from build123d import *

# Parameters (mm, degrees)
FILLET2_R               = 8
FILLET3_R               = 6
FILLET4_R               = 6
SKETCH3_R               = 10
CUT_EXTRUDE2_DEPTH      = 10
CUT_EXTRUDE2_DEPTH_BACK = 121
CHAMFER2_SIZE           = 6


with BuildPart() as part:
    # Sketch2 → Revolve1 (revolve)
    with BuildSketch(Plane.XY):
        Polygon((10, 120), (10, 0), (100, 0), (100, 20), (60, 20), (60, 60), (40, 60), (40, 120), align=None)
    revolve(axis=Axis((10, 120, 0), (0, -1, 0)))

    # Fillet2
    fillet2_edges = [part.edges().sort_by_distance(p)[0] for p in [
        (-80, 20, 0),
    ]]
    fillet(fillet2_edges, radius=FILLET2_R)

    # Fillet3
    fillet3_edges = [part.edges().sort_by_distance(p)[0] for p in [
        (-40, 20, 0),
    ]]
    fillet(fillet3_edges, radius=FILLET3_R)

    # Fillet4
    fillet4_edges = [part.edges().sort_by_distance(p)[0] for p in [
        (-20, 60, 0),
    ]]
    fillet(fillet4_edges, radius=FILLET4_R)

    # Sketch3 → Cut-Extrude2 (cut, two sides)
    with BuildSketch(Plane(origin=(0, 120, 0), x_dir=(1, 0, 0), z_dir=(0, 1, 0))) as cut_extrude2_sk:
        with Locations((10, 0)):
            Circle(SKETCH3_R)
    extrude(amount=CUT_EXTRUDE2_DEPTH, mode=Mode.SUBTRACT)
    extrude(cut_extrude2_sk.sketch, amount=-CUT_EXTRUDE2_DEPTH_BACK, mode=Mode.SUBTRACT)

    # Chamfer2
    chamfer2_edges = [part.edges().sort_by_distance(p)[0] for p in [
        (-20, 120, 0),
        (-40, 60, 0),
    ]]
    chamfer(chamfer2_edges, length=CHAMFER2_SIZE)


solid = part.part
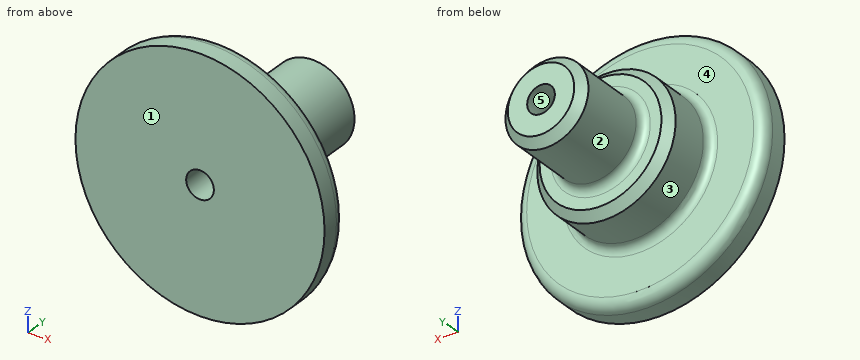
Input: part model. Units: mm. Frame: model coordinates. Face numbers are marked on the shaded views. A direction names the side the tool comes from. Give positions to 0.01 mm unless a question says otherwise; leave off trailing zeros. Loops run counter-clockwise (first coordinate to the right, second up) from the corner with the lowest first, then second, coordinate; pieces in that order, holes last. Notation, with made-up numbers: M -12,-11.5 L -4,-11.5 A16 ccw -4,-7.5 Z; hole C 89.25,71.5 d7. An arc over 180 degrees is marked long. Use CSV: the item, a comma, the result in double quotes.
(1) Material intervals for L1, parallel to Z at x = 10, y = 69; L2, parallel to Z at x = 10, y = 27; L3, parallel to Y at x = 50, z = 70.5, sorted ascending. Write a range as [from, to].
Outcome:
L1,"z = [-30, -10], [10, 30]"
L2,"z = [-50, -10], [10, 50]"
L3,"y = [0, 20]"
(2) Pull-direction query (X, two-part tool) for the marked faces 3, 4 and 5; classes: pulls with the +X half, pulls with the -X half, needs draft (parallel to the pull), parting line crosses it, or undercut.
Outcome:
face 3,"parting line crosses it"
face 4,"needs draft"
face 5,"undercut"
(3) Section A-A, the plane z = 0. Return loops of the section in (x, y).
Outcome:
outline,"M -80,0 L 0,0 L 0,120 L -14,120 L -20,114 L -20,66 A6 cw -26,60 L -34,60 L -40,54 L -40,26 A6 cw -46,20 L -72,20 A8 ccw -80,12 Z; M 20,0 L 100,0 L 100,12 A8 ccw 92,20 L 66,20 A6 cw 60,26 L 60,54 L 54,60 L 46,60 A6 cw 40,66 L 40,114 L 34,120 L 20,120 Z"
(4) Pin query (flat end, axial travel): P1, Ø4, axis at x = -25, y = 38, coming from the -Z side; P2, Ø5, axis at x = 35.5, z = -25, coming from the -Y side; P3, Ø10, axis at x = 50, z = 7.5, coming from the +Y side. Return the tip coordinate at first contact, or that it passes through.
Outcome:
P1,"stops at z = -37.56"
P2,"stops at y = 0"
P3,"stops at y = 60.01"
(5) Section D-D, the plane y = 17.5. Return loops of the section in (x, z).
Outcome:
outline,"C 10,0 d175.62; hole C 10,0 d20"
(6) Set-up query: the marked faces 1 and 2. Return all of +Z, -Z, +X, -X, +Y, -Y with unobstructed straight access to the full face (end or side cutting, diameter ignored); none if empty.
Outcome:
face 1,"+Z, -Z, +X, -X, -Y"
face 2,"+Y"
(7) Section C-C, the plane y = 104. Return loops of the section in (x, z), plus the area to 3 significant figures.
Outcome:
outline,"C 10,0 d60; hole C 10,0 d20"
area,"2,510 mm²"
(8) Section B-B, the plane x = 10. Return loops of the section in (y, z).
Outcome:
outline,"M 0,-90 L 12,-90 A8 ccw 20,-82 L 20,-56 A6 cw 26,-50 L 54,-50 L 60,-44 L 60,-36 A6 cw 66,-30 L 114,-30 L 120,-24 L 120,-10 L 0,-10 Z; M 0,10 L 120,10 L 120,24 L 114,30 L 66,30 A6 cw 60,36 L 60,44 L 54,50 L 26,50 A6 cw 20,56 L 20,82 A8 ccw 12,90 L 0,90 Z"
